from build123d import *

# Parameters (mm, degrees)
SKETCH1_R           = 20
SKETCH1_R_2         = 1.5
SKETCH1_R_3         = 1.65
BOSS_EXTRUDE2_DEPTH = 4
FILLET1_R           = 3


with BuildPart() as part:
    # Sketch1 → Boss-Extrude2 (new body)
    with BuildSketch(Plane(origin=(0, 0, 0), x_dir=(1, 0, 0), z_dir=(0, 1, 0))):
        Polygon((92.45867298, 93.85), (92.45867298, 53.803836873), (71.914755495, 50.55), (71.914755495, -50.55), (92.528223413, -53.3293777), (92.45867298, -93.85), (-18.04132702, -93.85), (-18.04132702, -160.15), (-59.04132702, -160.15), (-59.04132702, -93.85), (-177.54132702, -93.85), (-177.54132702, -32.5), (-184.54132702, -32.5), (-184.54132702, 32.5), (-177.54132702, 32.5), (-177.54132702, 34.274594508), (-177.54132702, 93.85), (-59.04132702, 93.85), (-59.04132702, 160.15), (-18.04132702, 160.15), (-18.04132702, 93.85), align=None)
        with Locations(Location((-47.54132702, 60, 0), (0, 0, 270))):
            Circle(SKETCH1_R, mode=Mode.SUBTRACT)
        with Locations(Location((-3.085244505, 0, 0), (0, 0, 270))):
            Circle(SKETCH1_R, mode=Mode.SUBTRACT)
        with Locations(Location((-47.54132702, -60, 0), (0, 0, 90))):
            Circle(SKETCH1_R, mode=Mode.SUBTRACT)
        with Locations(Location((-77.54132702, 77.85, 0), (0, 0, 270))):
            Circle(SKETCH1_R_2, mode=Mode.SUBTRACT)
        with Locations(Location((-121.62132702, 28.85, 0), (0, 0, 270))):
            Circle(SKETCH1_R_2, mode=Mode.SUBTRACT)
        with Locations(Location((-102.65132702, 28.85, 0), (0, 0, 270))):
            Circle(SKETCH1_R_2, mode=Mode.SUBTRACT)
        with Locations(Location((-121.62132702, -28.85, 0), (0, 0, 90))):
            Circle(SKETCH1_R_2, mode=Mode.SUBTRACT)
        with Locations(Location((-102.65132702, -28.85, 0), (0, 0, 90))):
            Circle(SKETCH1_R_2, mode=Mode.SUBTRACT)
        with Locations(Location((-77.54132702, -77.85, 0), (0, 0, 90))):
            Circle(SKETCH1_R_2, mode=Mode.SUBTRACT)
        with Locations(Location((37.024755495, 28.85, 0), (0, 0, 270))):
            Circle(SKETCH1_R_2, mode=Mode.SUBTRACT)
        with Locations(Location((12.45867298, 77.85, 0), (0, 0, 270))):
            Circle(SKETCH1_R_2, mode=Mode.SUBTRACT)
        with Locations(Location((-8.085244505, -58.85, 0), (0, 0, 270))):
            Circle(SKETCH1_R_2, mode=Mode.SUBTRACT)
        with Locations(Location((12.45867298, -77.85, 0), (0, 0, 90))):
            Circle(SKETCH1_R_2, mode=Mode.SUBTRACT)
        with Locations(Location((37.024755495, -28.85, 0), (0, 0, 90))):
            Circle(SKETCH1_R_2, mode=Mode.SUBTRACT)
        with Locations(Location((-121.62132702, -77.85, 0), (0, 0, 90))):
            Circle(SKETCH1_R_2, mode=Mode.SUBTRACT)
        with Locations(Location((-102.65132702, -77.85, 0), (0, 0, 90))):
            Circle(SKETCH1_R_2, mode=Mode.SUBTRACT)
        with Locations(Location((31.42867298, -77.85, 0), (0, 0, 90))):
            Circle(SKETCH1_R_2, mode=Mode.SUBTRACT)
        with Locations(Location((12.444755495, -28.85, 0), (0, 0, 90))):
            Circle(SKETCH1_R_2, mode=Mode.SUBTRACT)
        with Locations(Location((31.414755495, -28.85, 0), (0, 0, 90))):
            Circle(SKETCH1_R_2, mode=Mode.SUBTRACT)
        with Locations(Location((-121.62132702, 77.85, 0), (0, 0, 270))):
            Circle(SKETCH1_R_2, mode=Mode.SUBTRACT)
        with Locations(Location((-102.65132702, 77.85, 0), (0, 0, 270))):
            Circle(SKETCH1_R_2, mode=Mode.SUBTRACT)
        with Locations(Location((31.414755495, 28.85, 0), (0, 0, 270))):
            Circle(SKETCH1_R_2, mode=Mode.SUBTRACT)
        with Locations(Location((12.444755495, 28.85, 0), (0, 0, 270))):
            Circle(SKETCH1_R_2, mode=Mode.SUBTRACT)
        with Locations(Location((31.42867298, 77.85, 0), (0, 0, 270))):
            Circle(SKETCH1_R_2, mode=Mode.SUBTRACT)
        with Locations(Location((-47.54132702, -84, 0), (0, 0, 270))):
            Circle(SKETCH1_R_3, mode=Mode.SUBTRACT)
        with Locations(Location((-47.54132702, -36, 0), (0, 0, 270))):
            Circle(SKETCH1_R_3, mode=Mode.SUBTRACT)
        with Locations(Location((-3.085244505, -24, 0), (0, 0, 270))):
            Circle(SKETCH1_R_3, mode=Mode.SUBTRACT)
        with Locations(Location((-3.085244505, 24, 0), (0, 0, 270))):
            Circle(SKETCH1_R_3, mode=Mode.SUBTRACT)
        with Locations(Location((-47.54132702, 36, 0), (0, 0, 270))):
            Circle(SKETCH1_R_3, mode=Mode.SUBTRACT)
        with Locations(Location((-47.54132702, 84, 0), (0, 0, 270))):
            Circle(SKETCH1_R_3, mode=Mode.SUBTRACT)
    extrude(amount=BOSS_EXTRUDE2_DEPTH)

    # Fillet1
    fillet1_edges = [part.edges().sort_by_distance(p)[0] for p in [
        (-177.54132702, 2, -93.85),
        (-59.04132702, 2, -93.85),
        (-59.04132702, 2, -160.15),
        (-18.04132702, 2, -160.15),
        (-18.04132702, 2, -93.85),
        (92.45867298, 2, -93.85),
        (92.45867298, 2, -53.803836873),
        (71.914755495, 2, -50.55),
        (71.914755495, 2, 50.55),
        (92.528223413, 2, 53.3293777),
        (92.45867298, 2, 93.85),
        (-18.04132702, 2, 93.85),
        (-18.04132702, 2, 160.15),
        (-59.04132702, 2, 160.15),
        (-59.04132702, 2, 93.85),
        (-177.54132702, 2, 93.85),
        (-177.54132702, 2, 32.5),
        (-184.54132702, 2, 32.5),
        (-184.54132702, 2, -32.5),
        (-177.54132702, 2, -32.5),
    ]]
    fillet(fillet1_edges, radius=FILLET1_R)


solid = part.part
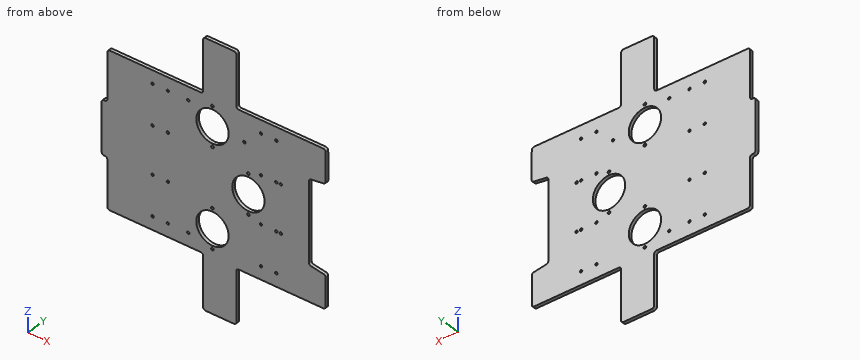
Source: CAD feature listing. Evaluate the final solid. Frame: model axes, mm. Give positions to 0.01 mm unless a question says otherwise; leave off trailing zeros. Order: outer loops, then holes, each group sorted by start corner. A loop starts at its lowest first (then second) coordinate and runs counter-clockwise, first axis right, second up. Notation, with made-up numbers: (35, 56.5) -> (71, 56.5) arc R18 ccw to (71, 86.5) -> close; hole circle Ø5 at (-28.5, 31). An arc over 180 degrees is marked (long way). Write item = value, one per line.
Item 1: Section query A-A (x = -31). Output: boundary loops of the cut face in (y, z).
Check result:
outline = (0, -160.15) -> (4, -160.15) -> (4, -71.24) -> (0, -71.24) -> close; (0, -48.76) -> (4, -48.76) -> (4, 48.76) -> (0, 48.76) -> close; (0, 71.24) -> (4, 71.24) -> (4, 160.15) -> (0, 160.15) -> close
Item 2: Section query B-B (z = 67). Output: boundary loops of the cut face in (x, y), then the cut area to 3 significant figures.
Check result:
outline = (-177.54, 0) -> (-66.28, 0) -> (-66.28, 4) -> (-177.54, 4) -> close; (-28.81, 0) -> (92.5, 0) -> (92.5, 4) -> (-28.81, 4) -> close
area = 930 mm²
Item 3: Section query D-D (x = -133.5). Output: boundary loops of the cut face in (y, z).
Check result:
outline = (0, -93.85) -> (4, -93.85) -> (4, 93.85) -> (0, 93.85) -> close
Item 4: Contact query for flat-ended pins moving along their axis: pin 1 (2 mm diameter, centred on y = 1, z = -94.5, fed in from +X); pin 2 (1.2 mm diameter, centred on y = 2.5, z = 133, fed in from +X); pin 3 (2 mm diameter, centred on y = 3.5, z = 122, fed in from -X). Output: stop coordinate, or through.
Check result:
pin_1 = 90.86
pin_2 = -18.04
pin_3 = -59.04
Item 5: Section query C-C (z = -115). Output: boundary loops of the cut face in (x, y), then the cut area to 3 significant figures.
Check result:
outline = (-59.04, 0) -> (-18.04, 0) -> (-18.04, 4) -> (-59.04, 4) -> close
area = 164 mm²
Item 6: Ray query, probe 1 along X at (y, z) = (1.2, -28.85); probe 2 along X at (y, z) = (2.9, -24.5); probe 3 along X at (y, z) = (0.25, 20.5). Return the intervals inside material, ascending.
Check result:
probe_1 = -184.54 to -123.12, -120.12 to -104.15, -101.15 to 10.94, 13.94 to 29.91, 32.91 to 35.52, 38.52 to 71.91
probe_2 = -184.54 to -4.66, -1.51 to 71.91
probe_3 = -184.54 to 71.91
